Here's how the part is built. I have some questions about the finished solid (model axes, mm). A direction names the side the tool comes from. Coordinates: 2 decimals unless noted, no trailing zeros. Write each loop counter-clockwise with the first axis right and the second up, starting at its lowest first coordinate (ties: lowest second). Pieces come first, ordered by that corner, then holes.
```python
from build123d import *

# Parameters (mm, degrees)
F0_W      = 120
F0_H      = 90
F1_DEPTH  = 2
F2_W      = 35
F2_H      = 47
F3_DEPTH  = 2
F5_D      = 3
F6_W      = 38
F6_H      = 60
F6_W_2    = 34
F6_H_2    = 56
F7_DEPTH  = 10
F8_W      = 34
F8_H      = 56
F9_DEPTH  = 12.001
F10_W     = 34
F10_H     = 56
F11_DEPTH = 2
F12_R     = 2
F13_DEPTH = 25


with BuildPart() as f1:
    # F0 (on Top) → F1 (new body)
    with BuildSketch(Plane.XY):
        with Locations((-20.18502, 10.433374)):
            Rectangle(F0_W, F0_H)
    extrude(amount=F1_DEPTH)

    # F2 (on face) → F3 (cut)
    with BuildSketch(Plane.XY.offset(2)):
        with Locations((-37.68502, 15.933374)):
            Rectangle(F2_W, F2_H)
    extrude(amount=-F3_DEPTH, mode=Mode.SUBTRACT)

    # F5 (through all)
    with Locations(Plane.XY.offset(2)):
        with Locations((-74.6, -29), (34.7, -29), (34.61498, 49.933374), (-74.68502, 49.933374)):
            Hole(F5_D / 2)

    # F6 (on face) → F7 (join)
    with BuildSketch(Plane.XY.offset(2)):
        with Locations((-0.18502, 15.433374)):
            Rectangle(F6_W, F6_H)
        with Locations((-0.18502, 15.433374)):
            Rectangle(F6_W_2, F6_H_2, mode=Mode.SUBTRACT)
        with Locations((-0.18502, 15.433374)):
            Rectangle(F6_W_2, F6_H_2)
    extrude(amount=F7_DEPTH)

    # F8 (on face) → F9 (cut, through all)
    with BuildSketch(Plane.XY.offset(12)):
        with Locations((-0.18502, 15.433374)):
            Rectangle(F8_W, F8_H)
    extrude(amount=-F9_DEPTH, mode=Mode.SUBTRACT)

    # F10 (on face) → F11 (join)
    with BuildSketch(Plane.XY.offset(12)):
        with Locations((-0.18502, 15.433374)):
            Rectangle(F10_W, F10_H)
    extrude(amount=-F11_DEPTH)

    # F12 (on face) → F13 (cut)
    with BuildSketch(Plane.XY.offset(2)):
        with Locations((-65.18502, 35.433374)):
            Circle(F12_R)
        with Locations((-65.18502, 20.433374)):
            Circle(F12_R)
        with Locations((-65.18502, 4.433374)):
            Circle(F12_R)
        with Locations((-61.18502, -17.182156)):
            Circle(F12_R)
        with Locations((-55.18502, -15.566626)):
            Circle(F12_R)
        with Locations((-43.226759, -16.566626)):
            Circle(F12_R)
        with Locations((-26.226759, -16.566626)):
            Circle(F12_R)
    extrude(amount=-F13_DEPTH, mode=Mode.SUBTRACT)


solid = f1.part
```
1) Imagine slicing it at B-B on y = -29. Please give me the cut outline in (x, z), then the cut area to 3 significant figures.
Values follow:
outline: (-80.19, 0) - (-76.1, 0) - (-76.1, 2) - (-80.19, 2) - close; (-73.1, 0) - (33.2, 0) - (33.2, 2) - (-73.1, 2) - close; (36.2, 0) - (39.81, 0) - (39.81, 2) - (36.2, 2) - close
area: 228 mm2
2) Imagine slicing it at C-C on x = -74.6. Please give me the cut outline in (y, z).
Values follow:
outline: (-34.57, 0) - (-30.5, 0) - (-30.5, 2) - (-34.57, 2) - close; (-27.5, 0) - (48.44, 0) - (48.44, 2) - (-27.5, 2) - close; (51.43, 0) - (55.43, 0) - (55.43, 2) - (51.43, 2) - close
3) Will these pins go through, and if not, where does the flat tip stop? pin 1 (4 mm diameter, centred on y = 32.5, z = 10.5, fed in from +X) (3 decimals); pin 2 (10 mm diameter, centred on x = -0.5, y = 16, fed in from -Z); pin 3 (3.5 mm diameter, centred on x = -65.19, y = 20.43, fed in from +Z); pin 4 (5 mm diameter, centred on x = 7.5, z = 5.5, fed in from -Y).
Values follow:
pin 1: stops at x = 18.815
pin 2: stops at z = 10
pin 3: passes through
pin 4: stops at y = -14.57
4) On a 3-axis mill with a long thin cutter (end or side, diameter ignored), from which of +Z, -Z, +X, -X, +Y, -Y can I reach the whole of each face in a straight line? I mean faces 1 (the face through (0, -14.567, 7)), 2 (the face through (0, 45.433, 7)), 3 (the face through (0, 43.433, 5)), 4 (the face through (18.815, 15, 7)). Say none if no direction works.
Values follow:
face 1: +Z, +X, -X, -Y
face 2: +Z, +X, -X, +Y
face 3: -Z
face 4: +Z, +X, +Y, -Y
5) We'd pull the mould along X, two halves only. Please class faces 5 (the face through (0, 16, 12)), 6 (the face through (33.23, 49.36, 0.99)), 7 (the face through (-19.185, 15, 7)): pulls with the +X half, pulls with the -X half, needs draft (parallel to the pull), parting line crosses it, or undercut.
Values follow:
face 5: needs draft
face 6: undercut
face 7: pulls with the -X half
6) Imagine slicing it at A-A on z = 5.75. Please give me the cut outline in (x, y).
Values follow:
outline: (-19.19, -14.57) - (18.81, -14.57) - (18.81, 45.43) - (-19.19, 45.43) - close; hole (-17.19, -12.57) - (16.81, -12.57) - (16.81, 43.43) - (-17.19, 43.43) - close
7) I need wall thicknesses on probe 1 along Y at (x, z) = (-48, 1); probe 2 along X at (y, z) = (40, 4.75); probe 3 along Y at (x, z) = (-74.6, 0.9). Which ranges of each line are inside material? Lowest first, please.
Values follow:
probe 1: y = -34.57 to -7.57, 39.43 to 55.43
probe 2: x = -19.19 to -17.19, 16.81 to 18.81
probe 3: y = -34.57 to -30.5, -27.5 to 48.44, 51.43 to 55.43
8) Imagine slicing it at D-D on x = 26. Please give me the cut outline in (y, z), then the cut area to 3 significant figures.
Values follow:
outline: (-34.57, 0) - (55.43, 0) - (55.43, 2) - (-34.57, 2) - close
area: 180 mm2
